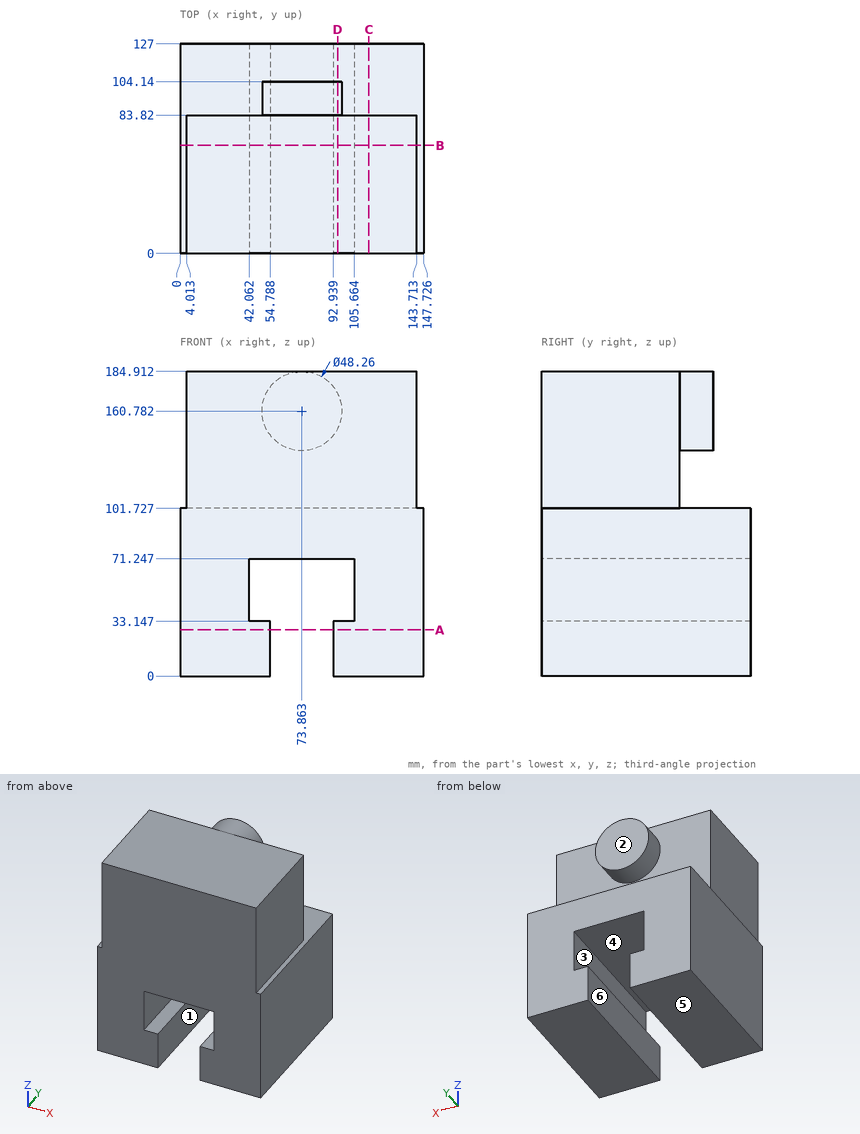
Source: three-view drawing plus pictorial views. Frame: mm from the lowest corner of the part. A direction names the side the tool comes from. Round coordinates to 2 decimals unless told otherwise and drop trailing zeros. Order: outer loops, then holes, each group sorted by start corner. A loop starts at its lowest first (then second) coordinate and runs counter-clockwise, first axis right, second up. Notation, with made-up numbers: (-11.75, 72) -> (15.25, 72) arc R26 ccw to (15.25, 96) -> close; hole circle Ø2 at (-23, 3). An arc over 180 degrees is marked (long way). Use CSV: the item, a comma, the result in double quotes. Start each with the question number.
1) Set-up query: the marked faces 1, 2 and 3. Return all of +Z, -Z, +X, -X, +Y, -Y with unobstructed straight access to the full face (end or side cutting, diameter ignored); none if empty.
2) Section A-A (z = 28). Return the cut outline in (x, y).
3) Draft query along Z for the marked faces 4, 5 and 6. Return one class per face: +Z half, -Z half, draft (parallel to the pull), parting line (faces both ways), or undercut.
4) Section C-C (x = 114.5). Return the cut outline in (y, z), and give its area (3 significant figures).
5) First-contact query: pin 1 Ø2 at (x, y) = (55.5, 90.5) entering from -Z; pin 2 Ø10 at (y, z) = (67.5, 141) entering from -X; pin 3 Ø5 at (x, z) = (68, 66.5) entering from +Y. Flat tips, straight axial feed; report the tip coordinate or a pass-through.
6) Section B-B (y = 65.5). Return the cut outline in (x, z).
7) Material intervals for line 1 along X through (y, z) = (95, 12.5); line 2 along X through (y, z) = (79, 70); line 3 along Z through (x, y) = (81, 11.5), sorted ascending. Write a range as from..to.
8) Section D-D (x = 95.5). Return the cut outline in (y, z), and give its area (3 significant figures).
Returned:
1,face 1,"-Z, +Y, -Y"
1,face 2,"+Z, +X, -X, +Y"
1,face 3,"+Y, -Y"
2,outline,"(0, 0) -> (54.79, 0) -> (54.79, 127) -> (0, 127) -> close; (92.94, 0) -> (147.73, 0) -> (147.73, 127) -> (92.94, 127) -> close"
3,face 4,"undercut"
3,face 5,"-Z half"
3,face 6,"draft"
4,outline,"(0, 0) -> (127, 0) -> (127, 101.73) -> (83.82, 101.73) -> (83.82, 184.91) -> (0, 184.91) -> close"
4,area,"19,900 mm²"
5,pin 1,"stops at z = 0"
5,pin 2,"stops at x = 4.01"
5,pin 3,"passes through"
6,outline,"(0, 0) -> (54.79, 0) -> (54.79, 33.15) -> (42.06, 33.15) -> (42.06, 71.25) -> (105.66, 71.25) -> (105.66, 33.15) -> (92.94, 33.15) -> (92.94, 0) -> (147.73, 0) -> (147.73, 101.73) -> (143.71, 101.73) -> (143.71, 184.91) -> (4.01, 184.91) -> (4.01, 101.73) -> (0, 101.73) -> close"
7,line 1,"x = 0..54.79, 92.94..147.73"
7,line 2,"x = 0..42.06, 105.66..147.73"
7,line 3,"z = 71.25..184.91"
8,outline,"(0, 0) -> (127, 0) -> (127, 33.15) -> (0, 33.15) -> close; (0, 71.25) -> (127, 71.25) -> (127, 101.73) -> (83.82, 101.73) -> (83.82, 150.1) -> (104.14, 150.1) -> (104.14, 171.46) -> (83.82, 171.46) -> (83.82, 184.91) -> (0, 184.91) -> close"
8,area,"15,500 mm²"
